Can you work these out from the model? Positions are in its coordinate system, mm. A direction names the side the tool comes from. Give positions to 0.01 mm unless a question says otherwise; leave off trailing zeros. Loops run counter-clockwise (first coordinate to the right, second up) from the corner with the lowest first, then second, coordinate; pieces in that order, holes last. Notation, with made-up numbers: (-13, 61) - (37, 61) arc R26 cw to (37, 82) - close; hole circle Ø1 at (-19, 3). An arc over 180 degrees is marked (long way). Answer in a Markdown table with one row per item.
Autodesk Inventor part; units mm, degrees
ref_plane "YZ Plane" through (0, 0, 0) normal (1, 0, 0) x (0, 1, 0)
ref_plane "XZ Plane" through (0, 0, 0) normal (0, 1, 0) x (-1, 0, 0)
ref_plane "XY Plane" through (0, 0, 0) normal (0, 0, 1) x (1, 0, 0)
sketch "Sketch1" plane through (0, 0, 0) normal (0, 0, 1) x (1, 0, 0)
  circle A0 centre (-43.950789, -25.375) radius 1.8
  circle A1 centre (0, -50.75) radius 1.8
  circle A2 centre (43.950789, -25.375) radius 1.8
  circle A3 centre (43.950789, 25.375) radius 1.8
  circle A4 centre (0, 50.75) radius 1.8
  circle A5 centre (-43.950789, 25.375) radius 1.8
  circle A6 centre (0, 0) radius 55
  circle A7 centre (0, 0) radius 10
  line L0 (-5, -45.365185) -> (-5, -28.788018)
  arc A8 (-3.318966, -27.298983) -> (-5, -28.788018) centre (-3.5, -28.788018) ccw
  arc A9 (-3.318966, -27.298983) -> (3.318966, -27.298983) centre (0, 0) ccw
  arc A10 (5, -28.788018) -> (3.318966, -27.298983) centre (3.5, -28.788018) ccw
  line L1 (5, -28.788018) -> (5, -45.365185)
  arc A11 (3.615385, -46.86074) -> (5, -45.365185) centre (3.5, -45.365185) ccw
  arc A12 (-3.615385, -46.86074) -> (3.615385, -46.86074) centre (0, 0) ccw
  arc A13 (-5, -45.365185) -> (-3.615385, -46.86074) centre (-3.5, -45.365185) ccw
  arc A14 (3.615385, 46.86074) -> (-3.615385, 46.86074) centre (0, 0) ccw
  arc A15 (5, 45.365185) -> (3.615385, 46.86074) centre (3.5, 45.365185) ccw
  line L2 (5, 45.365185) -> (5, 28.788018)
  arc A16 (3.318966, 27.298983) -> (5, 28.788018) centre (3.5, 28.788018) ccw
  arc A17 (3.318966, 27.298983) -> (-3.318966, 27.298983) centre (0, 0) ccw
  arc A18 (-5, 28.788018) -> (-3.318966, 27.298983) centre (-3.5, 28.788018) ccw
  line L3 (-5, 28.788018) -> (-5, 45.365185)
  arc A19 (-3.615385, 46.86074) -> (-5, 45.365185) centre (-3.5, 45.365185) ccw
  circle A20 centre (25.375, -43.950789) radius 3.75
  arc A21 (11.879121, -45.47402) -> (23.5, -40.703194) centre (0, 0) ccw
  arc A22 (10, -44.022721) -> (11.879121, -45.47402) centre (11.5, -44.022721) ccw
  line L4 (10, -44.022721) -> (10, -26.622359)
  arc A23 (10.905172, -25.24534) -> (10, -26.622359) centre (11.5, -26.622359) ccw
  arc A24 (10.905172, -25.24534) -> (25.24534, -10.905172) centre (0, 0) ccw
  arc A25 (26.622359, -10) -> (25.24534, -10.905172) centre (26.622359, -11.5) ccw
  line L5 (26.622359, -10) -> (44.022721, -10)
  arc A26 (45.47402, -11.879121) -> (44.022721, -10) centre (44.022721, -11.5) ccw
  arc A27 (23.5, -40.703194) -> (45.47402, -11.879121) centre (0, 0) ccw
  circle A28 centre (-50.75, 0) radius 3.75
  arc A29 (-46.86074, 3.615385) -> (-47, 0) centre (0, 0) ccw
  arc A30 (-45.365185, 5) -> (-46.86074, 3.615385) centre (-45.365185, 3.5) ccw
  line L6 (-45.365185, 5) -> (-28.788018, 5)
  arc A31 (-27.298983, 3.318966) -> (-28.788018, 5) centre (-28.788018, 3.5) ccw
  arc A32 (-27.298983, 3.318966) -> (-27.298983, -3.318966) centre (0, 0) ccw
  arc A33 (-28.788018, -5) -> (-27.298983, -3.318966) centre (-28.788018, -3.5) ccw
  line L7 (-28.788018, -5) -> (-45.365185, -5)
  arc A34 (-46.86074, -3.615385) -> (-45.365185, -5) centre (-45.365185, -3.5) ccw
  arc A35 (-47, 0) -> (-46.86074, -3.615385) centre (0, 0) ccw
  circle A36 centre (25.375, 43.950789) radius 3.75
  arc A37 (45.47402, 11.879121) -> (23.5, 40.703194) centre (0, 0) ccw
  arc A38 (44.022721, 10) -> (45.47402, 11.879121) centre (44.022721, 11.5) ccw
  line L8 (44.022721, 10) -> (26.622359, 10)
  arc A39 (25.24534, 10.905172) -> (26.622359, 10) centre (26.622359, 11.5) ccw
  arc A40 (25.24534, 10.905172) -> (10.905172, 25.24534) centre (0, 0) ccw
  arc A41 (10, 26.622359) -> (10.905172, 25.24534) centre (11.5, 26.622359) ccw
  line L9 (10, 26.622359) -> (10, 44.022721)
  arc A42 (11.879121, 45.47402) -> (10, 44.022721) centre (11.5, 44.022721) ccw
  arc A43 (23.5, 40.703194) -> (11.879121, 45.47402) centre (0, 0) ccw
  circle A44 centre (-25.375, 43.950789) radius 3.75
  arc A45 (-11.879121, 45.47402) -> (-23.5, 40.703194) centre (0, 0) ccw
  arc A46 (-10, 44.022721) -> (-11.879121, 45.47402) centre (-11.5, 44.022721) ccw
  line L10 (-10, 44.022721) -> (-10, 26.622359)
  arc A47 (-10.905172, 25.24534) -> (-10, 26.622359) centre (-11.5, 26.622359) ccw
  arc A48 (-10.905172, 25.24534) -> (-25.24534, 10.905172) centre (0, 0) ccw
  arc A49 (-26.622359, 10) -> (-25.24534, 10.905172) centre (-26.622359, 11.5) ccw
  line L11 (-26.622359, 10) -> (-44.022721, 10)
  arc A50 (-45.47402, 11.879121) -> (-44.022721, 10) centre (-44.022721, 11.5) ccw
  arc A51 (-23.5, 40.703194) -> (-45.47402, 11.879121) centre (0, 0) ccw
  circle A52 centre (-25.375, -43.950789) radius 3.75
  arc A53 (-45.47402, -11.879121) -> (-23.5, -40.703194) centre (0, 0) ccw
  arc A54 (-44.022721, -10) -> (-45.47402, -11.879121) centre (-44.022721, -11.5) ccw
  line L12 (-44.022721, -10) -> (-26.622359, -10)
  arc A55 (-25.24534, -10.905172) -> (-26.622359, -10) centre (-26.622359, -11.5) ccw
  arc A56 (-25.24534, -10.905172) -> (-10.905172, -25.24534) centre (0, 0) ccw
  arc A57 (-10, -26.622359) -> (-10.905172, -25.24534) centre (-11.5, -26.622359) ccw
  line L13 (-10, -26.622359) -> (-10, -44.022721)
  arc A58 (-11.879121, -45.47402) -> (-10, -44.022721) centre (-11.5, -44.022721) ccw
  arc A59 (-23.5, -40.703194) -> (-11.879121, -45.47402) centre (0, 0) ccw
  circle A60 centre (50.75, 0) radius 3.75
  arc A61 (46.86074, -3.615385) -> (47, 0) centre (0, 0) ccw
  arc A62 (45.365185, -5) -> (46.86074, -3.615385) centre (45.365185, -3.5) ccw
  line L14 (45.365185, -5) -> (28.788018, -5)
  arc A63 (27.298983, -3.318966) -> (28.788018, -5) centre (28.788018, -3.5) ccw
  arc A64 (27.298983, -3.318966) -> (27.298983, 3.318966) centre (0, 0) ccw
  arc A65 (28.788018, 5) -> (27.298983, 3.318966) centre (28.788018, 3.5) ccw
  line L15 (28.788018, 5) -> (45.365185, 5)
  arc A66 (46.86074, 3.615385) -> (45.365185, 5) centre (45.365185, 3.5) ccw
  arc A67 (47, 0) -> (46.86074, 3.615385) centre (0, 0) ccw
  circle A68 centre (-14.142136, -14.142136) radius 5
  circle A69 centre (14.142136, 14.142136) radius 5
  circle A70 centre (-14.142136, 14.142136) radius 5
  circle A71 centre (14.142136, -14.142136) radius 5
  circle A72 centre (0, 0) radius 27.5
  circle A73 centre (0, 20) radius 1.75
  circle A74 centre (-18.600039, -7.351092) radius 1.75
  circle A75 centre (18.59999, -7.351217) radius 1.75
  point P0 (0, 0)
  point P1 (-27.298983, -3.318966)
  point P2 (-25.24534, -10.905172)
  point P3 (-10.905172, -25.24534)
  point P4 (3.318966, -27.298983)
  point P5 (25.24534, -10.905172)
  point P6 (27.298983, 3.318966)
  point P7 (25.24534, 10.905172)
  point P8 (10.905172, 25.24534)
  point P9 (-3.318966, 27.298983)
  point P10 (-25.24534, 10.905172)
sketch "Sketch1 outline for Extrusion1" plane through (0, 0, 0) normal (0, 0, 1) x (1, 0, 0)
  arc A0 (-27.298983, -3.318966) -> (-25.24534, -10.905172) centre (0, 0) ccw
  arc A1 (-27.298983, 3.318966) -> (-27.298983, -3.318966) centre (0, 0) ccw
  arc A2 (-25.24534, -10.905172) -> (-10.905172, -25.24534) centre (0, 0) ccw
  arc A3 (-25.24534, 10.905172) -> (-27.298983, 3.318966) centre (0, 0) ccw
  arc A4 (-10.905172, -25.24534) -> (-3.318966, -27.298983) centre (0, 0) ccw
  arc A5 (-10.905172, 25.24534) -> (-25.24534, 10.905172) centre (0, 0) ccw
  arc A6 (-3.318966, -27.298983) -> (3.318966, -27.298983) centre (0, 0) ccw
  arc A7 (-3.318966, 27.298983) -> (-10.905172, 25.24534) centre (0, 0) ccw
  arc A8 (3.318966, -27.298983) -> (10.905172, -25.24534) centre (0, 0) ccw
  arc A9 (3.318966, 27.298983) -> (-3.318966, 27.298983) centre (0, 0) ccw
  arc A10 (10.905172, -25.24534) -> (25.24534, -10.905172) centre (0, 0) ccw
  arc A11 (10.905172, 25.24534) -> (3.318966, 27.298983) centre (0, 0) ccw
  arc A12 (25.24534, -10.905172) -> (27.298983, -3.318966) centre (0, 0) ccw
  arc A13 (25.24534, 10.905172) -> (10.905172, 25.24534) centre (0, 0) ccw
  arc A14 (27.298983, -3.318966) -> (27.298983, 3.318966) centre (0, 0) ccw
  arc A15 (27.298983, 3.318966) -> (25.24534, 10.905172) centre (0, 0) ccw
  circle A16 centre (-14.142136, -14.142136) radius 5
  circle A17 centre (-18.600039, -7.351092) radius 1.75
  circle A18 centre (14.142136, -14.142136) radius 5
  circle A19 centre (0, 0) radius 10
  circle A20 centre (18.59999, -7.351217) radius 1.75
  circle A21 centre (-14.142136, 14.142136) radius 5
  circle A22 centre (0, 20) radius 1.75
  circle A23 centre (14.142136, 14.142136) radius 5
extrude "Extrusion1" add sketch "Sketch1 outline for Extrusion1" along normal blind 3.175
sketch "Sketch2" plane through (0, 0, 3.175) normal (0, 0, 1) x (1, 0, 0)
  circle A0 centre (-23.0125, 0) radius 1.435
  circle A1 centre (23.0125, 0) radius 1.435
  point P0 (0, 0)
extrude "Extrusion2" cut sketch "Sketch2" against normal blind 3.175
sketch "Sketch3" plane through (0, 0, 0) normal (0, 0, -1) x (-1, 0, 0)
  circle A0 centre (-23.0125, 0) radius 1.435
  circle A1 centre (23.0125, 0) radius 1.435
  line L0 (-23.0125, 3.175426) -> (-20.2625, 1.587713)
  line L1 (-20.2625, 1.587713) -> (-20.2625, -1.587713)
  line L2 (-20.2625, -1.587713) -> (-23.0125, -3.175426)
  line L3 (-23.0125, -3.175426) -> (-25.7625, -1.587713)
  line L4 (-25.7625, -1.587713) -> (-25.7625, 1.587713)
  line L5 (-25.7625, 1.587713) -> (-23.0125, 3.175426)
  circle A2 centre (23.0125, 0) radius 1.435
  line L6 (23.0125, 3.175426) -> (25.7625, 1.587713)
  line L7 (25.7625, 1.587713) -> (25.7625, -1.587713)
  line L8 (25.7625, -1.587713) -> (23.0125, -3.175426)
  line L9 (23.0125, -3.175426) -> (20.2625, -1.587713)
  line L10 (20.2625, -1.587713) -> (20.2625, 1.587713)
  line L11 (20.2625, 1.587713) -> (23.0125, 3.175426)
  point P0 (0, 0)
  dimension "d4" = 5.5
  dimension "d5" = 5.5
extrude "Extrusion3" cut sketch "Sketch3" against normal blind 2.4
chamfer "Chamfer1" distance 0.5 angle 45 1 edges at (-25.2453, -10.9052, 3.175)
properties part number "AMT102Mount"
Q1. If I drill on line 1 (Y direction, x = 0, z = 1.1); line 2 (Y direction, x = 17.5, z = 2.1); line 3 (X direction, y = 11.5, z = 2.75), over which ranges is the centre line in solid material (lowest first)? Write a range as [from, to].
Checked values:
| item | result |
|---|---|
| line 1 | y = [-27.5, -10], [10, 18.25], [21.75, 27.5] |
| line 2 | y = [-21.21, -17.85], [-10.44, -8.71], [-5.99, 10.44], [17.85, 21.21] |
| line 3 | x = [-24.9, -18.39], [-9.9, 9.9], [18.39, 24.9] |
Q2. Imagine slicing it at B-B, the plane y = 0. Write out the boundary of the cut face in (x, z) (1 decimal), and give its area (3 significant figures).
Checked values:
| item | result |
|---|---|
| outline | (-27.5, 0) - (-25.8, 0) - (-25.8, 2.4) - (-24.4, 2.4) - (-24.4, 3.2) - (-27, 3.2) - (-27.5, 2.7) - close; (-21.6, 2.4) - (-20.3, 2.4) - (-20.3, 0) - (-10, 0) - (-10, 3.2) - (-21.6, 3.2) - close; (10, 0) - (20.3, 0) - (20.3, 2.4) - (21.6, 2.4) - (21.6, 3.2) - (10, 3.2) - close; (24.4, 2.4) - (25.8, 2.4) - (25.8, 0) - (27.5, 0) - (27.5, 2.7) - (27, 3.2) - (24.4, 3.2) - close |
| area | 80.0 mm² |
Q3. Imagine slicing it at A-A, the plane x = 0. Write out the boundary of the cut face in (y, z) (3 decimals).
Checked values:
| item | result |
|---|---|
| outline | (-27.5, 0) - (-10, 0) - (-10, 3.175) - (-27, 3.175) - (-27.5, 2.675) - close; (10, 0) - (18.25, 0) - (18.25, 3.175) - (10, 3.175) - close; (21.75, 0) - (27.5, 0) - (27.5, 2.675) - (27, 3.175) - (21.75, 3.175) - close |
Q4. On a 3-axis mill with a long thin cutter (end or side, diameter ignored), from which of +Z, -Z, +X, -X, +Y, -Y can I reach the whole of each face in a straight line? I mean faces 1 (the face through (-26.53, -7.24, 1.32)), 2 (the face through (-25.762, 0, 1)). Say none if no direction works.
Checked values:
| item | result |
|---|---|
| face 1 | +Z, -Z, -X, -Y |
| face 2 | -Z |
Q5. For pin 1 (9 mm diameter, centred on x = -14.14, y = -14.14, fed in from -Z); pin 2 (3.5 mm diameter, centred on x = 23.01, y = 0, fed in from -Z); pin 3 (0.7 mm diameter, centred on y = 0.5, z = 1.5, fed in from +X); pin 4 (1.5 mm diameter, centred on x = 12, z = 2.5, fed in from -Y), each with a flat end and sliding along its axis, tell me the tip position at first contact or that it passes through.
Checked values:
| item | result |
|---|---|
| pin 1 | passes through |
| pin 2 | stops at z = 2.4 |
| pin 3 | stops at x = 27.5 |
| pin 4 | stops at y = -25.09 |
Q6. Imagine slicing it at C-C, the plane z = 0.5. Count the separate pieces of the cut face and the enclosed holes in it, and give its area (3 significant figures).
Checked values:
| item | result |
|---|---|
| separate pieces | 1 |
| enclosed holes | 10 |
| area | 1,670 mm² |
Q7. If we mould it in two halves opening along Y, with no side actions, what happens to faces 3 (the face through (21.657, 2.393, 1.183)), 4 (the face through (-19.55, 19.34, 1.32)), 5 (the face through (-22.4, 1.5, 2.4)), 6 (the face through (-27.5, 0, 1.3))? For each: released by +Y, released by -Y, zero draft, split by the parting line, or undercut.
Checked values:
| item | result |
|---|---|
| face 3 | undercut |
| face 4 | released by +Y |
| face 5 | undercut |
| face 6 | split by the parting line |
